from build123d import *

# Parameters (mm, degrees)
F0_W          = 200
F0_H          = 100
F1_DEPTH      = 5
F2_W          = 30
F2_H          = 10
F3_DEPTH      = 30
F4_R          = 2.5
F5_DEPTH      = 100.001
F6_R          = 3
F6_R_2        = 2.5
F7_DEPTH      = 2
F7_DEPTH_BACK = 25
F8_R          = 3
F8_R_2        = 2.5
F9_DEPTH      = 2
F10_R         = 3
F10_R_2       = 2.5
F11_DEPTH     = 2
F12_R         = 3
F12_R_2       = 2.5
F13_DEPTH     = 2
F14_R         = 3
F14_R_2       = 2.5
F15_DEPTH     = 2
F16_R         = 3
F16_R_2       = 2.5
F17_DEPTH     = 2
F18_W         = 30
F18_H         = 5
F19_DEPTH     = 5
F20_R         = 1.25
F21_DEPTH     = 200.001
F22_R         = 2.49999
F23_W         = 30
F23_H         = 5
F24_DEPTH     = 5
F25_R         = 1.25
F26_DEPTH     = 200.001
F27_R         = 2.49999


# Not quite as in the source:
# - a fillet or chamfer is up to 0.001 mm smaller than in the source, because OpenCascade refuses the exact size


with BuildPart() as f1:
    # F0 (on Top) → F1 (new body)
    with BuildSketch(Plane.XY):
        with Locations((3.7896726225, 0)):
            Rectangle(F0_W, F0_H)
    extrude(amount=F1_DEPTH)

    # F2 (on face) → F3 (join)
    with BuildSketch(Plane.XY.offset(5)):
        with Locations((-81.2103273775, 45)):
            Rectangle(F2_W, F2_H)
        with Locations((88.7896726225, 45)):
            Rectangle(F2_W, F2_H)
        with Locations((-81.2103273775, -45)):
            Rectangle(F2_W, F2_H)
        with Locations((88.7896726225, -45)):
            Rectangle(F2_W, F2_H)
    extrude(amount=F3_DEPTH)

    # F4 (on face) → F5 (cut, through all)
    with BuildSketch(Plane.XZ.offset(50)):
        with Locations((88.7896726225, 20)):
            Circle(F4_R)
        with Locations((-81.2103273775, 20)):
            Circle(F4_R)
    extrude(amount=-F5_DEPTH, mode=Mode.SUBTRACT)

    # F6 (on face) → F7 (cut, two sides)
    with BuildSketch(Plane.XZ.offset(50)) as f7_sk:
        with Locations((88.7896726225, 20)):
            Circle(F6_R)
        with Locations((88.7896726225, 20)):
            Circle(F6_R_2, mode=Mode.SUBTRACT)
        with Locations((-81.2103273775, 20)):
            Circle(F6_R)
        with Locations((-81.2103273775, 20)):
            Circle(F6_R_2, mode=Mode.SUBTRACT)
    extrude(amount=-F7_DEPTH, mode=Mode.SUBTRACT)
    extrude(f7_sk.sketch, amount=F7_DEPTH_BACK, mode=Mode.SUBTRACT)

    # F8 (on face) → F9 (cut)
    with BuildSketch(Plane.XZ.offset(-40)):
        with Locations((-81.2103273775, 20)):
            Circle(F8_R)
        with Locations((-81.2103273775, 20)):
            Circle(F8_R_2, mode=Mode.SUBTRACT)
    extrude(amount=-F9_DEPTH, mode=Mode.SUBTRACT)

    # F10 (on face) → F11 (cut)
    with BuildSketch(Plane.XZ.offset(-40)):
        with Locations((88.7896726225, 20)):
            Circle(F10_R)
        with Locations((88.7896726225, 20)):
            Circle(F10_R_2, mode=Mode.SUBTRACT)
    extrude(amount=-F11_DEPTH, mode=Mode.SUBTRACT)

    # F12 (on face) → F13 (cut)
    with BuildSketch(Plane(origin=(0, 50, 0), x_dir=(-1, 0, 0), z_dir=(0, 1, 0))):
        with Locations((81.2103273775, 20)):
            Circle(F12_R)
        with Locations((81.2103273775, 20)):
            Circle(F12_R_2, mode=Mode.SUBTRACT)
        with Locations((-88.7896726225, 20)):
            Circle(F12_R)
        with Locations((-88.7896726225, 20)):
            Circle(F12_R_2, mode=Mode.SUBTRACT)
    extrude(amount=-F13_DEPTH, mode=Mode.SUBTRACT)

    # F14 (on face) → F15 (cut)
    with BuildSketch(Plane(origin=(0, -40, 0), x_dir=(-1, 0, 0), z_dir=(0, 1, 0))):
        with Locations((81.2103273775, 20)):
            Circle(F14_R)
        with Locations((81.2103273775, 20)):
            Circle(F14_R_2, mode=Mode.SUBTRACT)
        with Locations((81.2103273775, 20)):
            Circle(F14_R_2)
    extrude(amount=-F15_DEPTH, mode=Mode.SUBTRACT)

    # F16 (on face) → F17 (cut)
    with BuildSketch(Plane(origin=(0, -40, 0), x_dir=(-1, 0, 0), z_dir=(0, 1, 0))):
        with Locations((-88.7896726225, 20)):
            Circle(F16_R)
        with Locations((-88.7896726225, 20)):
            Circle(F16_R_2, mode=Mode.SUBTRACT)
    extrude(amount=-F17_DEPTH, mode=Mode.SUBTRACT)

    # F18 (on face) → F19 (join)
    with BuildSketch(Plane.XZ.offset(50)):
        with Locations((-81.2103273775, 2.5)):
            Rectangle(F18_W, F18_H)
        with Locations((88.7896726225, 2.5)):
            Rectangle(F18_W, F18_H)
    extrude(amount=F19_DEPTH)

    # F20 (on face) → F21 (cut, through all)
    with BuildSketch(Plane(origin=(-96.2103273775, 0, 0), x_dir=(0, -1, 0), z_dir=(-1, 0, 0))):
        with Locations((52.5, 2.5)):
            Circle(F20_R)
    extrude(amount=-F21_DEPTH, mode=Mode.SUBTRACT)

    # F22 (radius 2.5 in the source; OpenCascade refuses exactly that, so slightly less here)
    f22_edges = [f1.edges().sort_by_distance(p)[0] for p in [
        (-81.210327, -55, 5),
        (-81.210327, -55, 0),
        (88.789673, -55, 5),
        (88.789673, -55, 0),
    ]]
    fillet(f22_edges, radius=F22_R)

    # F23 (on face) → F24 (join)
    with BuildSketch(Plane(origin=(0, 50, 0), x_dir=(-1, 0, 0), z_dir=(0, 1, 0))):
        with Locations((-88.7896726225, 2.5)):
            Rectangle(F23_W, F23_H)
        with Locations((81.2103273775, 2.5)):
            Rectangle(F23_W, F23_H)
    extrude(amount=F24_DEPTH)

    # F25 (on face) → F26 (cut, through all)
    with BuildSketch(Plane(origin=(-96.2103273775, 0, 0), x_dir=(0, -1, 0), z_dir=(-1, 0, 0))):
        with Locations((-52.5, 2.5)):
            Circle(F25_R)
    extrude(amount=-F26_DEPTH, mode=Mode.SUBTRACT)

    # F27 (radius 2.5 in the source; OpenCascade refuses exactly that, so slightly less here)
    f27_edges = [f1.edges().sort_by_distance(p)[0] for p in [
        (88.789673, 55, 5),
        (88.789673, 55, 0),
        (-81.210327, 55, 0),
        (-81.210327, 55, 5),
    ]]
    fillet(f27_edges, radius=F27_R)


solid = f1.part
CAD build for the part. Positions are in the model's coordinates, mm. A direction names the side the tool comes from. Round coordinates to 2 decimals unless told otherwise and drop trailing zeros. Order: outer loops, then holes, each group sorted by start corner. A loop starts at its lowest first (then second) coordinate and runs counter-clockwise, first axis right, second up. Notation, with made-up numbers: (-26, 3) -> (-10, 3) arc R21 cw to (-10, 22) -> close; hole circle Ø5 at (7.5, 83.25). An arc over 180 degrees is marked (long way). Write item = value, one per line. Start each with the question number.
(1) Cut at C-C, the plane y = -36.5. List the corners of the cut face in (x, z), then the cut area to 3 significant figures.
(2) Pull direction X, two halves, no side cores. Call faces 1 (the flat face through (-66.21, 45, 20)), 2 (the flat face through (-96.21, -4, 4)), 3 (the flat face through (92, -40, 20)), 4 (the cylindrical face through (85.793, -49.014, 20.132)): released by +X, released by -X, zero draft, split by the parting line, or undercut.
(3) Which spindle directions (+Z, -Z, +X, -X, +Y, -Y) get a long thin tool onto all of the face, cutting with end or side? Do faces 5 (the flat face through (2, 1, 5)), 6 (the flat face through (92, 50, 20)), 7 (the flat face through (92, -50, 20)), 8 (the flat face through (87, -42, 22)). Say none if no direction does.
(4) Cut at B-B, the plane x = -58. List the corners of the cut face in (y, z).
(5) Cut at A-A, the plane z = 32.5. List the corners of the cut face in (x, y), then the cut area to 3 significant figures.
(6) Pin check, flat tips, straight feed: P1, Ø2.5, axis at y = 52, z = 3.5, coming from the +X side; P2, Ø1, axis at x = 77.5, y = 21, coming from the +Z side; P3, Ø9, axis at x = 82.5, z = 22, coming from the -Y side; P4, Ø3, axis at x = -82, z = 18.5, coming from the +Y side. Stop position of each tip, or through.
(7) Probe line 1 (Z direction, x = -73, y = -52.5); line 2 (X direction, y = 45, z = 28); line 3 (Y direction, x = -27.5, z = 2). List the from-to ranges inside material, lowest first. Write a range as [from, to].
Model answer:
q1.outline = (-96.21, 0) -> (103.79, 0) -> (103.79, 5) -> (-96.21, 5) -> close
q1.area = 1,000 mm2
q2.face_1 = undercut
q2.face_2 = released by -X
q2.face_3 = zero draft
q2.face_4 = undercut
q3.face_5 = +Z
q3.face_6 = +Z, +X, -X, +Y
q3.face_7 = +Z, +X, -X, -Y
q3.face_8 = none
q4.outline = (-50, 0) -> (50, 0) -> (50, 5) -> (-50, 5) -> close
q5.outline = (-96.21, -50) -> (-66.21, -50) -> (-66.21, -40) -> (-96.21, -40) -> close; (-96.21, 40) -> (-66.21, 40) -> (-66.21, 50) -> (-96.21, 50) -> close; (73.79, -50) -> (103.79, -50) -> (103.79, -40) -> (73.79, -40) -> close; (73.79, 40) -> (103.79, 40) -> (103.79, 50) -> (73.79, 50) -> close
q5.area = 1,200 mm2
q6.P1 = 103.79
q6.P2 = 5
q6.P3 = -50
q6.P4 = 50
q7.line_1 = [0, 1.25], [3.75, 5]
q7.line_2 = [-96.21, -66.21], [73.79, 103.79]
q7.line_3 = [-50, 50]
